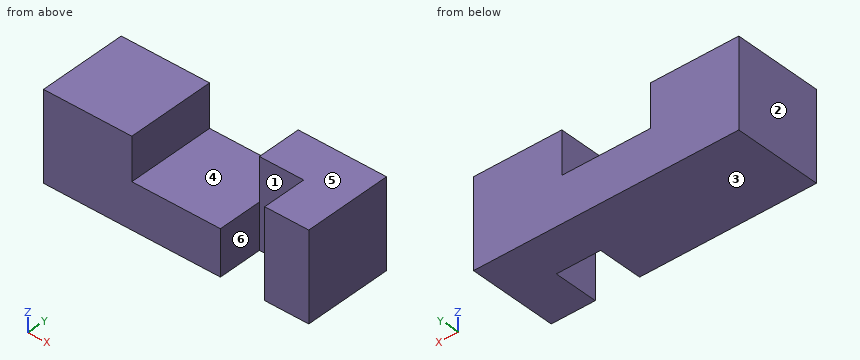
from build123d import *

# Parameters (mm, degrees)
F0_W     = 76.2
F0_H     = 25.4
F1_DEPTH = 25.4
F2_W     = 25.4508
F2_H     = 12.7254
F3_DEPTH = 25.4
F4_W     = 12.7254
F4_H     = 12.7254
F5_DEPTH = 25.4


with BuildPart() as f1:
    # F0 (on Top) → F1 (new body)
    with BuildSketch(Plane.XY):
        with Locations((38.1, 12.7)):
            Rectangle(F0_W, F0_H)
    extrude(amount=F1_DEPTH)

    # F2 (on Front) → F3 (cut)
    with BuildSketch(Plane.XZ):
        with Locations((38.1, 19.458432)):
            Rectangle(F2_W, F2_H)
    extrude(amount=-F3_DEPTH, mode=Mode.SUBTRACT)

    # F4 (on face) → F5 (cut)
    with BuildSketch(Plane.XY.offset(25.4)):
        with Locations((57.1881, 6.3627)):
            Rectangle(F4_W, F4_H)
    extrude(amount=-F5_DEPTH, mode=Mode.SUBTRACT)


solid = f1.part
Geometry: final body of the model. Coordinates: model frame, mm. Face numbers are marked on the shaded views. A direction names the side the tool comes from. Give positions to 0.01 mm unless a question says otherwise; leave off trailing zeros. Write each loop counter-clockwise with the first axis right and the second up, starting at its lowest first coordinate (ties: lowest second). Pieces come first, ordered by that corner, then holes. Notation, with made-up numbers: M 16,31.25 L 43,31.25 A29 cw 43,63.25 Z; hole C 45.5,81 d10. An arc over 180 degrees is marked long. Answer in a Markdown table with one row per item. Add a question column.
(1) Section D-D on y = 19.5. Return loops of the section in (x, z), and give its area (3 significant figures).
(2) Ray query, line 1 (X direction, y = 6, z = 17.75); line 2 (X direction, y = 11, z = 6.5); line 3 (Y direction, x = 61, z = 9.25). Return the intervals inside material, ascending.
(3) Section A-A on z = 18.75. Return loops of the section in (x, y).
(4) Mould query, pull axis X, two halves, no side actions, for the marked faces 1, 2 and 3. Classes: +X half, -X half, draft (parallel to the pull), parting line (faces both ways), or undercut.
(5) Section B-B on y = 11.25. Return loops of the section in (x, z).
(6) Section C-C on z = 12.25. Return loops of the section in (x, y), and give its area (3 significant figures).
(7) Reachability of the marked faces 4, 5 and 6 from +Z, -Z, +X, -X, +Y, -Y: full face, straight path, thin tool, end or side. Return the list, or none.
(8) First-contact query: pin 1 (8 mm diameter, centred on x = 45, z = 5.5, fed in from -Y); pin 2 (4 mm diameter, centred on x = 59, z = 9, fed in from -Y). Flat tips, straight axial feed; report the tip coordinate or a pass-through.
Result set:
| question | item | result |
|---|---|---|
| 1 | outline | M 0,0 L 76.2,0 L 76.2,25.4 L 50.83,25.4 L 50.83,13.1 L 25.37,13.1 L 25.37,25.4 L 0,25.4 Z |
| 1 | area | 1,620 mm^2 |
| 2 | line 1 | x = 0 to 25.37, 63.55 to 76.2 |
| 2 | line 2 | x = 0 to 50.83, 63.55 to 76.2 |
| 2 | line 3 | y = 12.73 to 25.4 |
| 3 | outline | M 0,0 L 25.37,0 L 25.37,25.4 L 0,25.4 Z; M 50.83,12.73 L 63.55,12.73 L 63.55,0 L 76.2,0 L 76.2,25.4 L 50.83,25.4 Z |
| 4 | face 1 | undercut |
| 4 | face 2 | -X half |
| 4 | face 3 | draft |
| 5 | outline | M 0,0 L 50.83,0 L 50.83,13.1 L 25.37,13.1 L 25.37,25.4 L 0,25.4 Z; M 63.55,0 L 76.2,0 L 76.2,25.4 L 63.55,25.4 Z |
| 6 | outline | M 0,0 L 50.83,0 L 50.83,12.73 L 63.55,12.73 L 63.55,0 L 76.2,0 L 76.2,25.4 L 0,25.4 Z |
| 6 | area | 1,770 mm^2 |
| 7 | face 4 | +Z, +Y, -Y |
| 7 | face 5 | +Z, +X, -X, +Y, -Y |
| 7 | face 6 | +Z, -Z, -Y |
| 8 | pin 1 | stops at y = 0 |
| 8 | pin 2 | stops at y = 12.73 |
